Geometry: final body of the model. Coordinates: model frame, mm. Give positions to 0.01 mm unless a question says otherwise; leave off trailing zeros. Write each loop counter-clockwise with the first axis right and the second up, starting at its lowest first coordinate (ties: lowest second). Pieces come first, ordered by that corner, then holes.
from build123d import *

# Parameters (mm, degrees)
SKETCH1_W               = 100
SKETCH1_H               = 100
BOSS_EXTRUDE1_DEPTH     = 10
CUT_EXTRUDE3_DEPTH      = 72.414284285
CUT_EXTRUDE3_DEPTH_BACK = 72.414284285
SKETCH3_R               = 10.025
SKETCH3_R_2             = 3.675


with BuildPart() as part:
    # Sketch1 → Boss-Extrude1 (new body)
    with BuildSketch(Plane(origin=(0, 0, 0), x_dir=(1, 0, 0), z_dir=(0, 1, 0))):
        Rectangle(SKETCH1_W, SKETCH1_H)
    extrude(amount=BOSS_EXTRUDE1_DEPTH)

    # Sketch3 → Cut-Extrude3 (cut, two sides: drawn at the far end of the back side and taken through both)
    with BuildSketch(Plane(origin=(0, 0, 0), x_dir=(1, 0, 0), z_dir=(0, 1, 0)).offset(-CUT_EXTRUDE3_DEPTH_BACK)):
        with Locations(Location((-32.7, 32.7, 0), (0, 0, 270))):
            Circle(SKETCH3_R)
        with Locations(Location((32.7, 32.7, 0), (0, 0, 270))):
            Circle(SKETCH3_R)
        with Locations(Location((32.7, -32.7, 0), (0, 0, 270))):
            Circle(SKETCH3_R)
        with Locations(Location((-32.7, -32.7, 0), (0, 0, 270))):
            Circle(SKETCH3_R)
        with Locations(Location((0, 32.7, 0), (0, 0, 270))):
            Circle(SKETCH3_R_2)
        with Locations(Location((32.7, 0, 0), (0, 0, 270))):
            Circle(SKETCH3_R_2)
        with Locations(Location((0, -32.7, 0), (0, 0, 270))):
            Circle(SKETCH3_R_2)
        with Locations(Location((-32.7, 0, 0), (0, 0, 270))):
            Circle(SKETCH3_R_2)
    extrude(amount=CUT_EXTRUDE3_DEPTH + CUT_EXTRUDE3_DEPTH_BACK, mode=Mode.SUBTRACT)


solid = part.part
Q1. Pull-direction query (Z, two-part tool) for faces 1 (the flat face through (-1, 5, 50)), 2 (the cylindrical face through (41.153, 4.93, 38.089)), 3 (the flat face through (-1, 0, -1)); classes: released by +Z, released by -Z, zero draft, split by the parting line, or undercut.
Filled sheet:
face 1: released by +Z
face 2: undercut
face 3: zero draft
Q2. Ray query, line 1 along Z through (x, y) = (0, 7) (3 decimals); line 2 along Z through (x, y) = (32.7, 4) (3 decimals). Return the intervals inside material, ascending.
Filled sheet:
line 1: z = -50 to -36.375, -29.025 to 29.025, 36.375 to 50
line 2: z = -50 to -42.725, -22.675 to -3.675, 3.675 to 22.675, 42.725 to 50
Q3. Section B-B on y = 7.5. Count the separate pieces of the cut face and the enclosed holes in it, plus the area to 3 significant figures.
Filled sheet:
separate pieces: 1
enclosed holes: 8
area: 8,570 mm2
Q4. Section D-D on z = -32.7. Output: boundary loops of the cut face in (x, y) (3 decimals).
Filled sheet:
outline: (-50, 0) - (-42.725, 0) - (-42.725, 10) - (-50, 10) - close; (-22.675, 0) - (-3.675, 0) - (-3.675, 10) - (-22.675, 10) - close; (3.675, 0) - (22.675, 0) - (22.675, 10) - (3.675, 10) - close; (42.725, 0) - (50, 0) - (50, 10) - (42.725, 10) - close
Q5. Pin query (flat end, axial travel): P1, Ø8.5, axis at x = 0, z = -32.7, coming from the -Y side. Return the tip coordinate at first contact, or that it passes through.
Filled sheet:
P1: stops at y = 0
Q6. Section A-A on z = 0. Output: boundary loops of the cut face in (x, y) (3 decimals), plus the area to 3 significant figures.
Filled sheet:
outline: (-50, 0) - (-36.375, 0) - (-36.375, 10) - (-50, 10) - close; (-29.025, 0) - (29.025, 0) - (29.025, 10) - (-29.025, 10) - close; (36.375, 0) - (50, 0) - (50, 10) - (36.375, 10) - close
area: 853 mm2
Q7. Section C-C on x = 32.7. Output: boundary loops of the cut face in (y, z) (3 decimals), plus the area to 4 significant figures.
Filled sheet:
outline: (0, -50) - (10, -50) - (10, -42.725) - (0, -42.725) - close; (0, -22.675) - (10, -22.675) - (10, -3.675) - (0, -3.675) - close; (0, 3.675) - (10, 3.675) - (10, 22.675) - (0, 22.675) - close; (0, 42.725) - (10, 42.725) - (10, 50) - (0, 50) - close
area: 525.5 mm2
